from build123d import *

# Parameters (mm, degrees)
EXTRUDE_1_DEPTH     = 3
SKETCH_2_R          = 1.575
SKETCH_2_R_2        = 6.75
SKETCH_2_R_3        = 1.6
SKETCH_2_W          = 10.2
SKETCH_2_H          = 20.2
CUT_EXTRUDE_1_DEPTH = 62.032778079
SKETCH_3_R          = 1
CUT_EXTRUDE_2_DEPTH = 62.032778079


with BuildPart() as part:
    # 草图1 → 凸台-拉伸1 (new body)
    with BuildSketch(Plane.XY):
        with BuildLine():
            Line((0, 0), (-46, 0))
            Line((-46, 0), (-46, -40))
            Line((-46, -40), (0, -40))
            ThreePointArc((0, -40), (20, -20), (0, 0))
        make_face()
    extrude(amount=EXTRUDE_1_DEPTH)

    # 草图2 → 切除-拉伸1 (cut, through all)
    with BuildSketch(Plane.XY.offset(3)):
        with Locations((-41, -15)):
            Circle(SKETCH_2_R)
        with Locations(Location((-41, -25, 0), (0, 0, 180))):
            Circle(SKETCH_2_R)
        with Locations((-21, -25)):
            Circle(SKETCH_2_R)
        with Locations(Location((-21, -15, 0), (0, 0, 180))):
            Circle(SKETCH_2_R)
        with Locations((5, -20)):
            Circle(SKETCH_2_R_2)
        with Locations((5, -10.5)):
            Circle(SKETCH_2_R_3)
        with Locations((13.227241336, -24.75)):
            Circle(SKETCH_2_R_3)
        with Locations((-3.227241336, -24.75)):
            Circle(SKETCH_2_R_3)
        with Locations((-31, -20)):
            Rectangle(SKETCH_2_W, SKETCH_2_H)
    extrude(amount=-CUT_EXTRUDE_1_DEPTH, mode=Mode.SUBTRACT)

    # 草图3 → 切除-拉伸2 (cut, through all)
    with BuildSketch(Plane.XY.offset(3)):
        with Locations((-25.9, -9.9)):
            Circle(SKETCH_3_R)
        with Locations((-25.9, -30.1)):
            Circle(SKETCH_3_R)
        with Locations((-36.1, -30.1)):
            Circle(SKETCH_3_R)
        with Locations((-36.1, -9.9)):
            Circle(SKETCH_3_R)
    extrude(amount=-CUT_EXTRUDE_2_DEPTH, mode=Mode.SUBTRACT)


solid = part.part
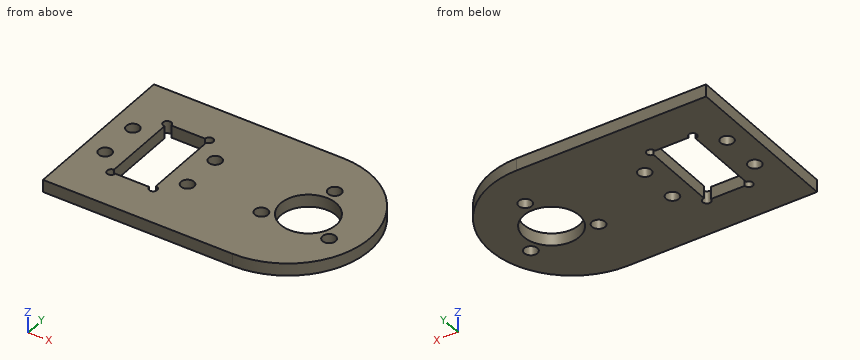
Work out the finished part from the listing and answer in its coordinate system (mm). Coordinates: 2 decimals unless noted, no trailing zeros. Write each loop counter-clockwise with the first axis right and the second up, starting at its lowest first coordinate (ties: lowest second). Pieces come first, ordered by that corner, then holes.
1. The part is cut by section A-A, the plane y = -20. Write down the section's boundary in (x, z).
Results list:
outline: (-46, 0) - (-36.1, 0) - (-36.1, 3) - (-46, 3) - close; (-25.9, 0) - (-1.75, 0) - (-1.75, 3) - (-25.9, 3) - close; (11.75, 0) - (20, 0) - (20, 3) - (11.75, 3) - close
2. A flat-ended cylindrical pin translates along its axis: pin 1 (2.5 mm diameter, centred on x = -36.1, y = -30.1, fed in from -Z). Find the tip coordinate at first contact, or state that the pin passes through.
Results list:
pin 1: stops at z = 0
3. The part is cut by section D-D, the plane x = 5. Write down the section's boundary in (y, z).
Results list:
outline: (-39.36, 0) - (-26.75, 0) - (-26.75, 3) - (-39.36, 3) - close; (-13.25, 0) - (-12.1, 0) - (-12.1, 3) - (-13.25, 3) - close; (-8.9, 0) - (-0.64, 0) - (-0.64, 3) - (-8.9, 3) - close
4. The part is cut by section B-B, the plane z = 1.3. State how many separate pieces and enclosed holes the cut face has, and give its area (3 significant figures).
Results list:
separate pieces: 1
enclosed holes: 9
area: 2,050 mm2
5. Consider line 1 along Y through (x, z) = (-41, 0.65) (3 decimals); line 2 along Y through (x, z) = (-37, 0.55); line 3 along X through (y, z) = (-30, 1). Determine where each line is inside the solid, lowest interval first.
Results list:
line 1: y = -40 to -26.575, -23.425 to -16.575, -13.425 to 0
line 2: y = -40 to -30.54, -29.66 to -10.34, -9.46 to 0
line 3: x = -46 to -37.09, -24.91 to 17.32
6. The part is cut by section C-C, the plane y = -15. Write down the section's boundary in (x, z) (3 decimals), and give its area (3 significant figures).
Results list:
outline: (-46, 0) - (-42.575, 0) - (-42.575, 3) - (-46, 3) - close; (-39.425, 0) - (-36.1, 0) - (-36.1, 3) - (-39.425, 3) - close; (-25.9, 0) - (-22.575, 0) - (-22.575, 3) - (-25.9, 3) - close; (-19.425, 0) - (0.465, 0) - (0.465, 3) - (-19.425, 3) - close; (9.535, 0) - (19.365, 0) - (19.365, 3) - (9.535, 3) - close
area: 119 mm2
